The model under review builds one solid part; all positions refer to its coordinate system, in mm. Face numbers are marked on the shaded views. A direction names the side the tool comes from. Give positions to 0.01 mm unless a question says otherwise; leave off trailing zeros. Loops run counter-clockwise (first coordinate to the right, second up) from the corner with the lowest first, then second, coordinate; pieces in that order, holes last. Notation, with made-up numbers: M 83.25,39.5 L 97.25,39.5 A15 cw 97.25,63.5 Z; hole C 39,-32.75 d7. An arc over 180 degrees is marked long. Return JSON: item names as keys, results as strings. Group by question number.
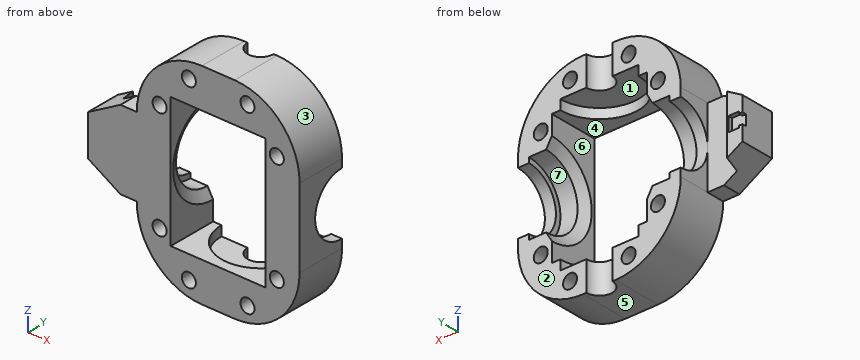
```python
from build123d import *
from OCP.BRepFilletAPI import BRepFilletAPI_MakeChamfer

# Parameters (mm, degrees)
SKETCH1_W           = 50
SKETCH1_H           = 64
SKETCH1_W_2         = 29.2
SKETCH1_H_2         = 40
BOSS_EXTRUDE1_DEPTH = 15
SKETCH3_W           = 7
SKETCH3_H           = 11.1
SKETCH4_R           = 9.5
CUT_EXTRUDE2_DEPTH  = 62.229078059
SKETCH5_R           = 4
CUT_EXTRUDE3_DEPTH  = 71.32780389
SKETCH8_R           = 2.15
CUT_EXTRUDE6_DEPTH  = 44.289721644
FILLET1_R           = 20
CHAMFER1_SIZE       = 3
CHAMFER1_SIZE2      = 1.732050808
SKETCH9_W           = 12
SKETCH9_H           = 3
SKETCH10_W          = 24
SKETCH10_H          = 5.5
BOSS_EXTRUDE2_DEPTH = 15
BOSS_EXTRUDE3_START = 9
SKETCH12_W          = 24
SKETCH12_H          = 3.7
BOSS_EXTRUDE3_DEPTH = 6
BOSS_EXTRUDE4_DEPTH = 1.3
CHAMFER2_SIZE2      = 1.339745962
CHAMFER2_SIZE       = 5
CHAMFER3_SIZE       = 10
CHAMFER3_SIZE2      = 5.773502692


with BuildPart() as part:
    # Sketch1 → Boss-Extrude1 (new body)
    with BuildSketch(Plane(origin=(0, 0, 0), x_dir=(1, 0, 0), z_dir=(0, 1, 0))):
        Rectangle(SKETCH1_W, SKETCH1_H)
        Rectangle(SKETCH1_W_2, SKETCH1_H_2, mode=Mode.SUBTRACT)
    extrude(amount=BOSS_EXTRUDE1_DEPTH)

    # Sketch3 → Cut-Revolve1 (revolve, cut)
    with BuildSketch(Plane(origin=(0, 15, 0), x_dir=(1, 0, 0), z_dir=(0, 1, 0))):
        with Locations((18.1, -5.55)):
            Rectangle(SKETCH3_W, SKETCH3_H)
        with Locations((-18.1, -5.55)):
            Rectangle(SKETCH3_W, SKETCH3_H)
    revolve(axis=Axis((14.6, 15, 0), (1, 0, 0)), mode=Mode.SUBTRACT)

    # Sketch4 → Cut-Extrude2 (cut, through all)
    with BuildSketch(Plane(origin=(25, 0, 0), x_dir=(0, 0, -1), z_dir=(1, 0, 0))):
        with Locations((0, 15)):
            Circle(SKETCH4_R)
    extrude(amount=-CUT_EXTRUDE2_DEPTH, mode=Mode.SUBTRACT)

    # Sketch5 → Cut-Extrude3 (cut, through all)
    with BuildSketch(Plane.XY.offset(32)):
        with Locations((0, 15)):
            Circle(SKETCH5_R)
    extrude(amount=-CUT_EXTRUDE3_DEPTH, mode=Mode.SUBTRACT)

    # Sketch8 → Cut-Extrude6 (cut, through all)
    with BuildSketch(Plane(origin=(0, 15, 0), x_dir=(1, 0, 0), z_dir=(0, 1, 0))):
        with Locations(Location((18, 16.5, 0), (0, 0, 270))):
            Circle(SKETCH8_R)
        with Locations(Location((18, -16.5, 0), (0, 0, 270))):
            Circle(SKETCH8_R)
        with Locations(Location((-18, -16.5, 0), (0, 0, 270))):
            Circle(SKETCH8_R)
        with Locations(Location((-18, 16.5, 0), (0, 0, 270))):
            Circle(SKETCH8_R)
        with Locations(Location((9, -27, 0), (0, 0, 270))):
            Circle(SKETCH8_R)
        with Locations(Location((-9, -27, 0), (0, 0, 270))):
            Circle(SKETCH8_R)
        with Locations(Location((-9, 27, 0), (0, 0, 270))):
            Circle(SKETCH8_R)
        with Locations(Location((9, 27, 0), (0, 0, 270))):
            Circle(SKETCH8_R)
    extrude(amount=-CUT_EXTRUDE6_DEPTH, mode=Mode.SUBTRACT)

    # Fillet1
    fillet1_edges = [part.edges().sort_by_distance(p)[0] for p in [
        (-25, 7.5, -32),
        (25, 7.5, -32),
        (25, 7.5, 32),
        (-25, 7.5, 32),
    ]]
    fillet(fillet1_edges, radius=FILLET1_R)

    # Chamfer1: one chamfer whose edges measure the first distance from different faces: ONE call of the kernel's chamfer builder (chamfer() names one face for all edges)
    chamfer1_edges_1 = [part.edges().sort_by_distance(p)[0] for p in [
        (14.6, 3.9, 0),
    ]]
    chamfer1_side_1 = [part.faces().sort_by_distance(p)[0] for p in [
        (14.6, 0.427200187, 0),
    ]]
    chamfer1_edges_2 = [part.edges().sort_by_distance(p)[0] for p in [
        (-14.6, 3.9, 0),
    ]]
    chamfer1_side_2 = [part.faces().sort_by_distance(p)[0] for p in [
        (-14.6, 0.427200187, 0),
    ]]
    chamfer1 = BRepFilletAPI_MakeChamfer(part.part.solid().wrapped)
    for e in chamfer1_edges_1:
        chamfer1.Add(CHAMFER1_SIZE, CHAMFER1_SIZE2, e.wrapped, chamfer1_side_1[0].wrapped)  # the first distance lies on this face
    for e in chamfer1_edges_2:
        chamfer1.Add(CHAMFER1_SIZE, CHAMFER1_SIZE2, e.wrapped, chamfer1_side_2[0].wrapped)  # the first distance lies on this face
    add(Compound.cast(chamfer1.Shape()), mode=Mode.REPLACE)

    # Sketch9 → Cut-Revolve2 (revolve, cut)
    with BuildSketch(Plane(origin=(0, 15, 0), x_dir=(1, 0, 0), z_dir=(0, 1, 0))):
        with Locations((-6, -21.5)):
            Rectangle(SKETCH9_W, SKETCH9_H)
        with Locations((-6, 21.5)):
            Rectangle(SKETCH9_W, SKETCH9_H)
    revolve(axis=Axis((0, 15, -29.871415895), (0, 0, 1)), mode=Mode.SUBTRACT)

    # Sketch10 → Boss-Extrude2 (add)
    with BuildSketch(Plane.ZY.offset(25)):
        with Locations((0, 2.75)):
            Rectangle(SKETCH10_W, SKETCH10_H)
    extrude(amount=BOSS_EXTRUDE2_DEPTH)

    # Sketch12 → Boss-Extrude3 (add)
    with BuildSketch(Plane.ZY.offset(25).offset(BOSS_EXTRUDE3_START)):
        with Locations((0, 7.35)):
            Rectangle(SKETCH12_W, SKETCH12_H)
    extrude(amount=BOSS_EXTRUDE3_DEPTH)

    # Sketch13 → Boss-Extrude4 (add)
    with BuildSketch(Plane(origin=(0, 9.2, 0), x_dir=(1, 0, 0), z_dir=(0, 1, 0))):
        Polygon((-38.9, 2.2), (-38.9, 1.6), (-40, 1.6), (-40, 12), (-34, 12), (-34, -12), (-40, -12), (-40, -1.6), (-38.9, -1.6), (-38.9, -2.2), (-35.7, -2.2), (-35.7, 2.2), align=None)
    extrude(amount=BOSS_EXTRUDE4_DEPTH)

    # Chamfer2
    chamfer2_edges = [part.edges().sort_by_distance(p)[0] for p in [
        (-34, 10.5, 0),
    ]]
    chamfer2_side = [part.faces().sort_by_distance(p)[0] for p in [
        (-34, 10.473205081, 0),
    ]]
    chamfer(chamfer2_edges, length=CHAMFER2_SIZE - 0.0001, length2=CHAMFER2_SIZE2 - 0.0001, reference=chamfer2_side[0])  # a hair under: the kernel refuses the full size

    # Chamfer3: one chamfer whose edges measure the first distance from different faces: ONE call of the kernel's chamfer builder (chamfer() names one face for all edges)
    chamfer3_edges_1 = [part.edges().sort_by_distance(p)[0] for p in [
        (-40, 5.25, 12),
    ]]
    chamfer3_side_1 = [part.faces().sort_by_distance(p)[0] for p in [
        (-33.677093858, 4.00630158, 12),
    ]]
    chamfer3_edges_2 = [part.edges().sort_by_distance(p)[0] for p in [
        (-40, 5.25, -12),
    ]]
    chamfer3_side_2 = [part.faces().sort_by_distance(p)[0] for p in [
        (-33.677093858, 4.00630158, -12),
    ]]
    chamfer3 = BRepFilletAPI_MakeChamfer(part.part.solid().wrapped)
    for e in chamfer3_edges_1:
        chamfer3.Add(CHAMFER3_SIZE, CHAMFER3_SIZE2, e.wrapped, chamfer3_side_1[0].wrapped)  # the first distance lies on this face
    for e in chamfer3_edges_2:
        chamfer3.Add(CHAMFER3_SIZE, CHAMFER3_SIZE2, e.wrapped, chamfer3_side_2[0].wrapped)  # the first distance lies on this face
    add(Compound.cast(chamfer3.Shape()), mode=Mode.REPLACE)


solid = part.part
```
(1) Add section D-D (x = 18). Write out the cut boundary in (y, z), and give its area (3 significant figures).
(2) Add section C-C (z = -27). Write out the cut boundary in (x, y).
(3) For the marked faces 5, 6 and 7, list the 3-axis set-ups (+Z, -Z, +X, -X, +Y, -Y) from which the entire face can be reached by the end or side of a thin tool; tool diameter is ignored.
(4) For probe 1 along Z at (x, y) = (4, 11.5); probe 2 along X at (y, z) = (7.5, 27); probe 3 along X at (y, z) = (1.5, -6), list the stretches that pass through material, from the lowest coordinate up.
(5) Add section A-A (x = 0). Write out the cut boundary in (y, z), and give its area (3 significant figures).
(6) For pin 1 (8 mm diameter, centred on x = 17.5, y = 10.5, fed in from +Z); pin 2 (4 mm diameter, centred on x = 9.5, y = 3.5, fed in from -Z); pin 3 (1.5 mm diameter, centred on x = -32, z = -5, fed in from +Y), all flat-tipped, find the tip position at first contact; note any pin that passes through.
(7) Add section B-B (x = -8). Write out the cut boundary in (y, z).
(8) Mouldability with a two-part tool opening along X and no side actions: class the marked faces 1, 2, 3 and 4 as released by +X, released by -X, zero draft, split by the parting line, or undercut.
Verdict:
{
 "1": {"outline": "M 0,-27.2 L 15,-27.2 L 15,-18.65 L 0,-18.65 Z; M 0,-14.35 L 15,-14.35 L 15,-11.1 A11.1 cw 15,11.1 L 15,14.35 L 0,14.35 Z; M 0,18.65 L 15,18.65 L 15,27.2 L 0,27.2 Z", "area": "493 mm²"},
 "2": {"outline": "M -18.23,0 L -11.15,0 L -11.15,15 L -18.23,15 Z; M -6.85,0 L 6.85,0 L 6.85,15 L 4,15 A4 cw -4,15 L -6.85,15 Z; M 11.15,0 L 18.23,0 L 18.23,15 L 11.15,15 Z"},
 "3": {"face 5": "-Z, +X, -X, +Y, -Y", "face 6": "+Y, -Y", "face 7": "+Y"},
 "4": {"probe 1": "z = -32 to -23, 23 to 32", "probe 2": "x = -18.23 to -11.15, -6.85 to 6.85, 11.15 to 18.23", "probe 3": "x = -40 to -14.6, 14.6 to 25"},
 "5": {"outline": "M 0,-32 L 11,-32 L 11,-23 L 3,-23 L 3,-20 L 0,-20 Z; M 0,20 L 3,20 L 3,23 L 11,23 L 11,32 L 0,32 Z", "area": "216 mm²"},
 "6": {"pin 1": "stops at z = 30.1", "pin 2": "stops at z = -31.84", "pin 3": "stops at y = 5.5"},
 "7": {"outline": "M 0,-31.77 L 15,-31.77 L 15,-28.9 L 0,-28.9 Z; M 0,-25.1 L 15,-25.1 L 15,-23 L 6.06,-23 L 6.06,-20 L 0,-20 Z; M 0,20 L 6.06,20 L 6.06,23 L 15,23 L 15,25.1 L 0,25.1 Z; M 0,28.9 L 15,28.9 L 15,31.77 L 0,31.77 Z"},
 "8": {"face 1": "undercut", "face 2": "zero draft", "face 3": "released by +X", "face 4": "undercut"}
}
